from build123d import *

# Parameters (mm, degrees)
SKETCH1_W           = 5
SKETCH1_H           = 5
BOSS_EXTRUDE1_DEPTH = 5
SKETCH2_R           = 1.05
CUT_EXTRUDE1_DEPTH  = 3
CUT_EXTRUDE2_START  = -3
SKETCH3_R           = 1.05
CUT_EXTRUDE2_DEPTH  = 3


with BuildPart() as part:
    # Sketch1 → Boss-Extrude1 (new, symmetric)
    with BuildSketch(Plane(origin=(0, 0, 0), x_dir=(1, 0, 0), z_dir=(0, 1, 0))):
        Rectangle(SKETCH1_W, SKETCH1_H)
    extrude(amount=BOSS_EXTRUDE1_DEPTH, both=True)

    # Sketch2 → Cut-Extrude1 (cut)
    with BuildSketch(Plane(origin=(0, 5, 0), x_dir=(1, 0, 0), z_dir=(0, 1, 0))):
        with Locations(Location((0, 0, 0), (0, 0, 270))):
            Circle(SKETCH2_R)
    extrude(amount=-CUT_EXTRUDE1_DEPTH, mode=Mode.SUBTRACT)

    # Sketch3 → Cut-Extrude2 (cut)
    with BuildSketch(Plane.XZ.offset(5).offset(CUT_EXTRUDE2_START)):
        with Locations(Location((0, 0, 0), (0, 0, 90))):
            Circle(SKETCH3_R)
    extrude(amount=CUT_EXTRUDE2_DEPTH, mode=Mode.SUBTRACT)


solid = part.part
Could you check a few things on this model? Use its own coordinates, in mm. A direction names the side the tool comes from. Give positions to 0.01 mm unless a question says otherwise; leave off trailing zeros. Order: outer loops, then holes, each group sorted by start corner. A loop starts at its lowest first (then second) coordinate and runs counter-clockwise, first axis right, second up.
Item 1: If we mould it in two halves opening along X, with no side actions, what happens to faces 1 (the face through (0, 0, 2.5)), 2 (the face through (-0.32, -3.48, 1)), 3 (the face through (-2.5, 0, 0))? For each: pulls with the +X half, pulls with the -X half, needs draft (parallel to the pull), parting line crosses it, or undercut.
Item 2: If we section it at B-B, the plane y = 3.5: Write out the boundary of the cut face in (x, z).
Item 3: For faces 4 (the face through (2.5, 0, 0)), 5 (the face through (0, 2, 0)), 6 (the face through (0, -2, 0)), which set-ups out of +Z, -Z, +X, -X, +Y, -Y let a thin tool reach every point of the face, with its end or its side?
Item 4: If we section it at A-A, the plane x = 0: Write out the boundary of the cut face in (y, z), plus the area to 3 significant figures.
Item 5: I'm going to push flat-ended pins straight in: pin 1 (1.7 mm diameter, centred on x = 0, z = 0, fed in from +Y); pin 2 (1 mm diameter, centred on x = 0.5, z = 0, fed in from -Y). Where does each tip first touch, or does it pass through?
Item 6: I need wall thicknesses on line 1 (X direction, y = 3.15, z = 0); line 2 (Y direction, x = -0.35, z = -0.6); line 3 (Z direction, x = 0.45, y = -2.25). Which ranges of each line are inside material? Lowest first, please.
Item 7: If we section it at C-C, the plane z = 0: Write out the boundary of the cut face in (x, y).
Values:
1. face 1: needs draft
1. face 2: undercut
1. face 3: pulls with the -X half
2. outline: (-2.5, -2.5) - (2.5, -2.5) - (2.5, 2.5) - (-2.5, 2.5) - close; hole circle Ø2.1 at (0, 0)
3. face 4: +Z, -Z, +X, +Y, -Y
3. face 5: +Y
3. face 6: -Y
4. outline: (-5, -2.5) - (5, -2.5) - (5, -1.05) - (2, -1.05) - (2, 1.05) - (5, 1.05) - (5, 2.5) - (-5, 2.5) - (-5, 1.05) - (-2, 1.05) - (-2, -1.05) - (-5, -1.05) - close
4. area: 37.4 mm2
5. pin 1: stops at y = 2
5. pin 2: stops at y = -2
6. line 1: x = -2.5 to -1.05, 1.05 to 2.5
6. line 2: y = -2 to 2
6. line 3: z = -2.5 to -0.95, 0.95 to 2.5
7. outline: (-2.5, -5) - (-1.05, -5) - (-1.05, -2) - (1.05, -2) - (1.05, -5) - (2.5, -5) - (2.5, 5) - (1.05, 5) - (1.05, 2) - (-1.05, 2) - (-1.05, 5) - (-2.5, 5) - close
